Read the model definition and answer for the solid it produces. Units are mm, in the model's axes. Face numbers are marked on the shaded views. A direction names the side the tool comes from. Round coordinates to 2 decimals unless told otherwise and drop trailing zeros. Write each loop counter-clockwise with the first axis right and the second up, starting at its lowest first coordinate (ties: lowest second). Pieces come first, ordered by that corner, then holes. Notation, with made-up numbers: (43.25, 44) - (55.25, 44) arc R14 cw to (55.25, 58) - close; hole circle Ø7 at (7, 52.5). An arc over 180 degrees is marked (long way). One line per item, written item: value. Start each with the question number.
(1) The mould has two halves that part along X. Classify the marked faces 1, 2 and 3: +X half, -X half, draft (parallel to the pull), parting line (faces both ways), or undercut.
(2) A cutting plane is placed at D-D, the plane z = -5.5. Determine the outline of the cut face in (x, y).
(3) Find the intervals of material crossed by L1, parallel to X at y = 4, z = -6.5; L2, parallel to Y at x = -3.25, z = 0; L3, parallel to Y at x = -5, z = 0, in increasing order.
(4) Flat-ended cylindrical pins translate along their axes: pin 1 Ø5 at (y, z) = (-3.5, 2.5) entering from +X; pin 2 Ø3 at (x, y) = (-3, 6) entering from +Z; pin 3 Ø1.5 at (x, y) = (-2.5, -3) entering from +Z; pin 4 Ø3 at (x, y) = (-11, -5.5) entering from +Z. Find the tip coordinate at first contact, or state that the pin passes through.
(5) For the marked faces 4 and 5, determine the directions among +Z, -Z, +X, -X, +Y, -Y from which every point of the face is accessible in a straight line to the end or side of a thin tool.
(6) A cutting plane is placed at C-C, the plane x = -2.75. Determine the outline of the cut face in (y, z).
(7) A cutting plane is placed at A-A, the plane z = 0. Determine the outline of the cut face in (x, y).
from build123d import *

# Parameters (mm, degrees)
SKETCH1_R           = 8
BOSS_EXTRUDE1_DEPTH = 13
SKETCH4_R           = 2.1
CUT_EXTRUDE1_DEPTH  = 18.23368794
FILLET1_R           = 0.5
SKETCH2_W           = 6
SKETCH2_H           = 2


with BuildPart() as part:
    # Sketch1 → Boss-Extrude1 (new body)
    with BuildSketch(Plane(origin=(0, 0, 0), x_dir=(0, 0, -1), z_dir=(1, 0, 0))):
        Circle(SKETCH1_R)
    extrude(amount=-BOSS_EXTRUDE1_DEPTH)

    # Sketch4 → Cut-Extrude1 (cut, through all)
    with BuildSketch(Plane(origin=(0, 0, 0), x_dir=(0, 0, -1), z_dir=(1, 0, 0))):
        Circle(SKETCH4_R)
    extrude(amount=-CUT_EXTRUDE1_DEPTH, mode=Mode.SUBTRACT)

    # Fillet1
    fillet1_edges = [part.edges().sort_by_distance(p)[0] for p in [
        (-13, 0, 2.1),
        (0, 0, 2.1),
    ]]
    fillet(fillet1_edges, radius=FILLET1_R)

    # Sketch2 → Cut-Revolve1 (revolve, cut)
    with BuildSketch(Plane.XY, mode=Mode.PRIVATE) as cut_revolve1_sk:
        with Locations((-6.7, 7)):
            Rectangle(SKETCH2_W, SKETCH2_H)
    revolve(cut_revolve1_sk.sketch.rotate(Axis((-13, 0, 0), (1, 0, 0)), 270), axis=Axis((-13, 0, 0), (1, 0, 0)), mode=Mode.SUBTRACT)


solid = part.part
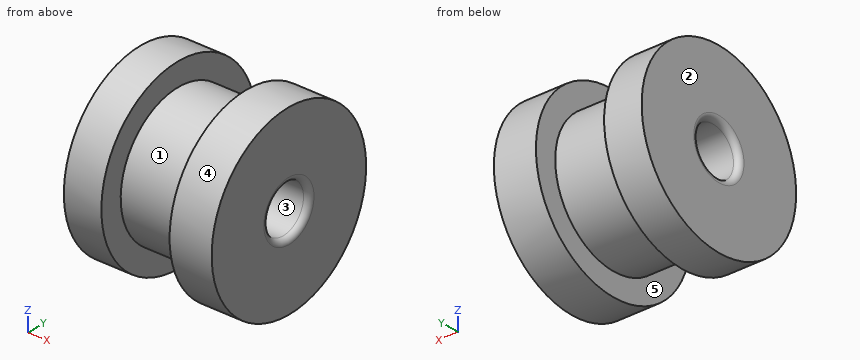
Here are the results:
1. face 1: undercut
1. face 2: -X half
1. face 3: draft
2. outline: (-13, -5.81) - (-9.7, -5.81) - (-9.7, -2.4) - (-3.7, -2.4) - (-3.7, -5.81) - (0, -5.81) - (0, 5.81) - (-3.7, 5.81) - (-3.7, 2.4) - (-9.7, 2.4) - (-9.7, 5.81) - (-13, 5.81) - close
3. L1: -13 to -9.7, -3.7 to 0
3. L2: -8 to -2.1, 2.1 to 8
3. L3: -6 to -2.1, 2.1 to 6
4. pin 1: x = 0
4. pin 2: z = 6.61
4. pin 3: z = 7.68
4. pin 4: z = 6.93
5. face 4: +X, -X
5. face 5: none
6. outline: circle Ø16 at (0, 0); hole circle Ø4.2 at (0, 0)
7. outline: (-13, -8) - (-9.7, -8) - (-9.7, -6) - (-3.7, -6) - (-3.7, -8) - (0, -8) - (0, -2.6) arc R0.5 ccw to (-0.5, -2.1) - (-12.5, -2.1) arc R0.5 ccw to (-13, -2.6) - close; (-13, 2.6) arc R0.5 ccw to (-12.5, 2.1) - (-0.5, 2.1) arc R0.5 ccw to (0, 2.6) - (0, 8) - (-3.7, 8) - (-3.7, 6) - (-9.7, 6) - (-9.7, 8) - (-13, 8) - close
